The drawing under review shows one solid part. Ordinate dimensions are in mm from its lowest x, y, z. Coordinates: 2 decimals unless noted, no trailing zeros. Loops run counter-clockwise (first coordinate to the right, second up) from the corner with the lowest first, then second, coordinate; pieces in that order, holes last. Notation, with made-up numbers: (75, 18.5) - (107, 18.5) arc R13 cw to (107, 37.5) - close; hole circle Ø4 at (14, 34). An arc over 180 degrees is marked (long way). Use one line per item in the form item = value. Start each with the question number.
1. To check wall thickness, follow probe 1 along X at (y, z) = (4, 4.2); probe 2 along Y at (x, z) = (2.5, 2.3) (3 decimals); probe 3 along X at (y, z) = (2, 3.9). State the ranges of each line that lie inside material, in increasing order.
2. Add section B-B on z = 4. Give the boundary of the cut face in (x, y) (3 decimals).
3. Add section A-A on y = 3.5. Give the boundary of the cut face in (x, z) (3 decimals).
4. Draft analysis for pull direction X (two halves, no side actions). For the marked faces 1, 2 and 3, state which applies: +X half, -X half, draft (parallel to the pull), parting line (faces both ways), or undercut.
5. Add section D-D on y = 6.5. Give the boundary of the cut face in (x, z), and give its area (3 significant figures).
6. Add section C-C on x = 42.5. Give the boundary of the cut face in (y, z) (3 decimals).
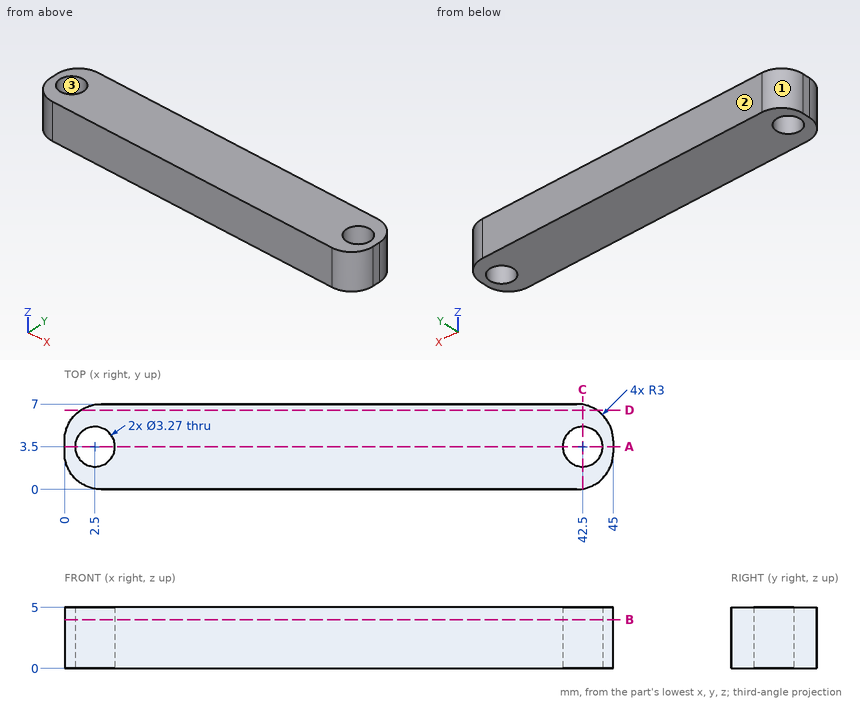
Conclusion:
q1.probe_1 = 0 to 0.94, 4.06 to 40.94, 44.06 to 45
q1.probe_2 = 0.042 to 1.865, 5.135 to 6.958
q1.probe_3 = 0.17 to 1.85, 3.15 to 41.85, 43.15 to 44.83
q2.outline = (0, 3) arc R3 ccw to (3, 0) - (42, 0) arc R3 ccw to (45, 3) - (45, 4) arc R3 ccw to (42, 7) - (3, 7) arc R3 ccw to (0, 4) - close; hole circle Ø3.27 at (2.5, 3.5); hole circle Ø3.27 at (42.5, 3.5)
q3.outline = (0, 0) - (0.865, 0) - (0.865, 5) - (0, 5) - close; (4.135, 0) - (40.865, 0) - (40.865, 5) - (4.135, 5) - close; (44.135, 0) - (45, 0) - (45, 5) - (44.135, 5) - close
q4.face_1 = -X half
q4.face_2 = draft
q4.face_3 = undercut
q5.outline = (1.34, 0) - (43.66, 0) - (43.66, 5) - (1.34, 5) - close
q5.area = 212 mm^2
q6.outline = (0.042, 0) - (1.865, 0) - (1.865, 5) - (0.042, 5) - close; (5.135, 0) - (6.958, 0) - (6.958, 5) - (5.135, 5) - close
